Geometry check sheet. Reference: the model listing, model coordinates, mm. Face numbers are marked on the shaded views. A direction names the side the tool comes from. Coordinates: 2 decimals unless noted, no trailing zeros. Loops run counter-clockwise (first coordinate to the right, second up) from the corner with the lowest first, then second, coordinate; pieces in that order, holes last.
from build123d import *

# Parameters (mm, degrees)
SKETCH1_R               = 53
BOSS_EXTRUDE2_DEPTH     = 45
SKETCH2_R               = 50.25
CUT_EXTRUDE1_DEPTH      = 39
SKETCH4_R               = 22
CUT_EXTRUDE3_DEPTH      = 39
BOSS_EXTRUDE3_START     = 8
BOSS_EXTRUDE3_DEPTH     = 8
CUT_EXTRUDE5_DEPTH      = 10
CUT_EXTRUDE5_DEPTH_BACK = 10
SKETCH10_R              = 1.5
BOSS_EXTRUDE6_START     = -8
BOSS_EXTRUDE6_DEPTH     = 16
SKETCH13_W              = 8
SKETCH13_H              = 16
BOSS_EXTRUDE7_DEPTH     = 14
FILLET1_R               = 8
LPATTERN1_COUNT         = 4
LPATTERN1_PITCH         = 14
FILLET1_OF_LPATTERN1_R  = 8
CUT_EXTRUDE6_DEPTH      = 119.482066153
CUT_EXTRUDE6_DEPTH_BACK = 119.482066153
SKETCH14_R              = 2


# Read off the part's stored shape, not the designer's step: Boss-Extrude6
with BuildPart() as part:
    # Sketch1 → Boss-Extrude2 (new body)
    with BuildSketch(Plane.XY):
        with Locations(Location((0, 0, 0), (0, 0, 180))):
            Circle(SKETCH1_R)
    extrude(amount=BOSS_EXTRUDE2_DEPTH)

    # Sketch2 → Cut-Extrude1 (cut)
    with BuildSketch(Plane.XY.offset(45)):
        Circle(SKETCH2_R)
    extrude(amount=-CUT_EXTRUDE1_DEPTH, mode=Mode.SUBTRACT)

    # Sketch4 → Cut-Extrude3 (cut)
    with BuildSketch(Plane(origin=(0, 0, 0), x_dir=(-1, 0, 0), z_dir=(0, 0, -1))):
        Circle(SKETCH4_R)
    extrude(amount=-CUT_EXTRUDE3_DEPTH, mode=Mode.SUBTRACT)

    # Sketch5 → Boss-Extrude3 (add)
    with BuildSketch(Plane(origin=(0, 0, 0), x_dir=(-1, 0, 0), z_dir=(0, 0, -1)).offset(BOSS_EXTRUDE3_START)):
        with BuildLine():
            Line((19.052558883, 11), (51.845925587, 11))
            ThreePointArc((51.845925587, 11), (10.588828865, 51.931461594), (-43.400241675, 30.42070056))
            Line((-43.400241675, 30.42070056), (-16.397830673, 14.666667965))
            ThreePointArc((-16.397830673, 14.666667965), (2.263406494, 21.883258236), (19.052558883, 11))
        make_face()
    extrude(amount=-BOSS_EXTRUDE3_DEPTH)

    # Sketch10 → Cut-Extrude5 (cut, two sides: drawn at the far end of the back side and taken through both)
    with BuildSketch(Plane(origin=(0, 0, 0), x_dir=(-1, 0, 0), z_dir=(0, 0, -1)).offset(-CUT_EXTRUDE5_DEPTH_BACK)):
        with Locations(Location((-39.35, -16.057007816, 0), (0, 0, 180))):
            Circle(SKETCH10_R)
        with Locations(Location((-39.178670952, 16.470632727, 0), (0, 0, 180))):
            Circle(SKETCH10_R)
        with Locations(Location((-16.057007816, 39.35, 0), (0, 0, 180))):
            Circle(SKETCH10_R)
        with Locations(Location((16.470632727, 39.178670952, 0), (0, 0, 180))):
            Circle(SKETCH10_R)
        with Locations(Location((39.35, 16.057007816, 0), (0, 0, 180))):
            Circle(SKETCH10_R)
        with Locations(Location((39.178670952, -16.470632727, 0), (0, 0, 180))):
            Circle(SKETCH10_R)
        with Locations(Location((16.057007816, -39.35, 0), (0, 0, 180))):
            Circle(SKETCH10_R)
        with Locations(Location((-16.470632728, -39.178670952, 0), (0, 0, 180))):
            Circle(SKETCH10_R)
    extrude(amount=CUT_EXTRUDE5_DEPTH + CUT_EXTRUDE5_DEPTH_BACK, mode=Mode.SUBTRACT)

    # Boss-Extrude6 outline → Boss-Extrude6 (add)
    with BuildSketch(Plane.XY.offset(BOSS_EXTRUDE6_START)):
        with BuildLine():
            Line((-25, 63), (-25, 46.733285782))
            ThreePointArc((-25, 46.733285782), (0, 53), (25, 46.733285782))
            Line((25, 46.733285782), (25, 63))
            Line((25, 63), (-25, 63))
        make_face()
    extrude(amount=BOSS_EXTRUDE6_DEPTH)

    # Sketch13 → Boss-Extrude7 (add)
    with BuildSketch(Plane(origin=(0, 63, 0), x_dir=(1, 0, 0), z_dir=(0, 1, 0))):
        with Locations((21, 0)):
            Rectangle(SKETCH13_W, SKETCH13_H)
    boss_extrude7 = extrude(amount=BOSS_EXTRUDE7_DEPTH)

    # Fillet1
    fillet1_edges = [part.edges().sort_by_distance(p)[0] for p in [
        (21, 77, 8),
        (21, 77, -8),
    ]]
    fillet(fillet1_edges, radius=FILLET1_R - 0.0001)  # a hair under: the kernel refuses the full size

    # LPattern1: Boss-Extrude7 ×4
    with Locations(*[(-i * LPATTERN1_PITCH, 0, 0) for i in range(1, LPATTERN1_COUNT)]):
        add(boss_extrude7)

    # Fillet1 of LPattern1
    fillet1_of_lpattern1_edges = [part.edges().sort_by_distance(p)[0] for p in [
        (7, 77, 8),
        (7, 77, -8),
        (-7, 77, 8),
        (-7, 77, -8),
        (-21, 77, 8),
        (-21, 77, -8),
    ]]
    fillet(fillet1_of_lpattern1_edges, radius=FILLET1_OF_LPATTERN1_R - 0.0001)  # a hair under: the kernel refuses the full size

    # Sketch14 → Cut-Extrude6 (cut, two sides: drawn at the far end of the back side and taken through both)
    with BuildSketch(Plane(origin=(25, 0, 0), x_dir=(0, 0, -1), z_dir=(1, 0, 0)).offset(-CUT_EXTRUDE6_DEPTH_BACK)):
        with Locations((0, 69)):
            Circle(SKETCH14_R)
    extrude(amount=CUT_EXTRUDE6_DEPTH + CUT_EXTRUDE6_DEPTH_BACK, mode=Mode.SUBTRACT)


solid = part.part
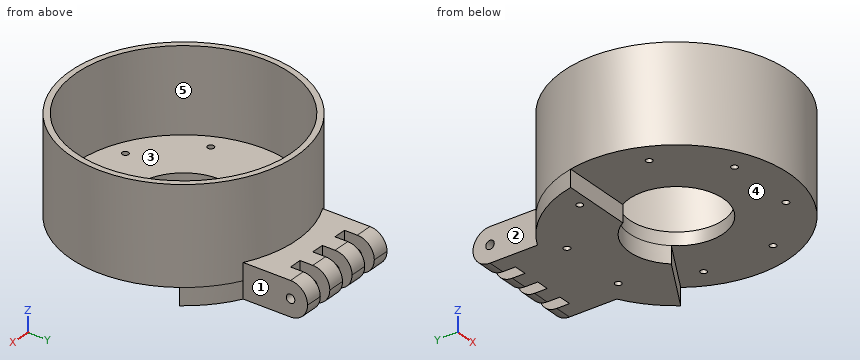
1) Section check A-A on x = 0. Record the cut outline in (y, z), and give its area (4 significant figures).
Data:
outline: (-53, 0) - (-22, 0) - (-22, 6) - (-50.25, 6) - (-50.25, 45) - (-53, 45) - close; (22, -8) - (63, -8) - (63, 8) - (53, 8) - (53, 45) - (50.25, 45) - (50.25, 6) - (22, 6) - close
area: 994.5 mm2
2) Material ranges on probe 1 along X at (y, z) = (69.5, -5.5); probe 2 along Y at (x, z) = (0, 17); probe 3 along Z at (x, y) = (8, 69), recorded low to high.
Data:
probe 1: x = -25 to -17, -11 to -3, 3 to 11, 17 to 25
probe 2: y = -53 to -50.25, 50.25 to 53
probe 3: z = -8 to -2, 2 to 8
3) Section check B-B on z = 37.5. Record the cut outline in (x, y).
Data:
outline: circle Ø106 at (0, 0); hole circle Ø100.5 at (0, 0)
4) Access from +Z, -Z, +X, -X, +Y, -Y to the whole of each face (thin tool, end or side, straight path). Record for the marked faces 1, 2 and 3.
Data:
face 1: +Z, -Z, +X, +Y
face 2: +Z, -Z, -X, +Y
face 3: +Z
5) Depth check by flat-ended pin: pin 1 (7 mm diameter, centred on y = 67, z = -3.5, fed in from -X); pin 2 (5 mm diameter, centred on y = 48.5, z = 39.5, fed in from -X); pin 3 (5 mm diameter, centred on x = -37, z = 19, fed in from -Y). Enter the tip coordinate at first touch or a pass-through.
Data:
pin 1: stops at x = -25
pin 2: stops at x = -26.32
pin 3: stops at y = -40.23
6) Mould release check, pull along Y, two halves, no side actions. Record for the marked faces 4 and 5: +Y half, -Y half, draft (parallel to the pull), parting line (faces both ways), or undercut.
Data:
face 4: draft
face 5: undercut
7) Section check C-C on x = 30. Record the cut outline in (y, z), and give its area (3 significant figures).
Data:
outline: (-43.69, 0) - (22.6, 0) - (22.6, -8) - (43.69, -8) - (43.69, 45) - (40.31, 45) - (40.31, 6) - (-40.31, 6) - (-40.31, 45) - (-43.69, 45) - close
area: 957 mm2
8) Section check D-D on y = 56. Record the cut outline in (x, z).
Data:
outline: (-25, -8) - (25, -8) - (25, 8) - (-25, 8) - close
